from build123d import *

# Parameters (mm, degrees)
ESQUISSE1_R           = 9
BOSS_EXTRU_1_DEPTH    = 5
ESQUISSE1_R_2         = 25.075
ESQUISSE1_R_3         = 23.6
BOSS_EXTRU_1_2_DEPTH  = 5
ESQUISSE1_3_R         = 23.6
ESQUISSE1_3_R_2       = 9
BOSS_EXTRU_2_DEPTH    = 2
ESQUISSE1_4_R         = 29.5
ESQUISSE1_4_R_2       = 25.075
BOSS_EXTRU_3_DEPTH    = 5.1
CONG_1_R              = 2
CONG_1_OF_SYM_TRIE1_R = 2


with BuildPart() as part:
    # Esquisse1 → Boss.-Extru.1 (new body)
    with BuildSketch(Plane.XY):
        Circle(ESQUISSE1_R)
        with BuildLine():
            ThreePointArc((-3, 0), (2.001193394, -2.235), (0.33015, 2.981778157))
            Line((0.33015, 2.981778157), (-3, 0))
        make_face(mode=Mode.SUBTRACT)
    boss_extru_1 = extrude(amount=BOSS_EXTRU_1_DEPTH)



with BuildPart() as body_2:
    # Esquisse1 → Boss.-Extru.1 2 (new body)
    with BuildSketch(Plane.XY):
        Circle(ESQUISSE1_R_2)
        Circle(ESQUISSE1_R_3, mode=Mode.SUBTRACT)
    boss_extru_1_2 = extrude(amount=BOSS_EXTRU_1_2_DEPTH)


with BuildPart() as part_1:
    add(part.part)

    add(body_2.part)  # Boss.-Extru.2 merges body 2
    # Esquisse1<3> → Boss.-Extru.2 (add)
    with BuildSketch(Plane.XY):
        Circle(ESQUISSE1_3_R)
        Circle(ESQUISSE1_3_R_2, mode=Mode.SUBTRACT)
    boss_extru_2 = extrude(amount=BOSS_EXTRU_2_DEPTH)

    # Esquisse1<4> → Boss.-Extru.3 (add)
    with BuildSketch(Plane.XY):
        Circle(ESQUISSE1_4_R)
        Circle(ESQUISSE1_4_R_2, mode=Mode.SUBTRACT)
    boss_extru_3 = extrude(amount=BOSS_EXTRU_3_DEPTH)

    # Congé1
    cong_1_edges = [part_1.edges().sort_by_distance(p)[0] for p in [
        (-9, 0, 2),
        (-23.6, 0, 2),
    ]]
    fillet(cong_1_edges, radius=CONG_1_R)


with BuildPart() as sym_trie1_1:
    # Symétrie1: Boss.-Extru.1, Boss.-Extru.1 2, Boss.-Extru.2, Boss.-Extru.3 across Front Plane
    add(boss_extru_1.mirror(Plane.XY))
    add(boss_extru_1_2.mirror(Plane.XY))
    add(boss_extru_2.mirror(Plane.XY))
    add(boss_extru_3.mirror(Plane.XY))

    # Congé1 of Symétrie1
    cong_1_of_sym_trie1_edges = [sym_trie1_1.edges().sort_by_distance(p)[0] for p in [
        (-9, 0, -2),
        (-23.6, 0, -2),
    ]]
    fillet(cong_1_of_sym_trie1_edges, radius=CONG_1_OF_SYM_TRIE1_R)


with BuildPart() as part_2:
    add(part_1.part)

    # Symétrie1 united with what the copies to: union Symétrie1_1
    add(sym_trie1_1.part)


solid = part_2.part
Design review of the part built by this model. Coordinates are the model's own, in mm. A direction names the side the tool comes from. Coordinates: 2 decimals unless noted, no trailing zeros. Write each loop counter-clockwise with the first axis right and the second up, starting at its lowest first coordinate (ties: lowest second). Pieces come first, ordered by that corner, then holes. Notation, with made-up numbers: (23, -39.75) - (41, -39.75) arc R6 cw to (41, -32.75) - close; hole circle Ø3 at (-33, 55). An arc over 180 degrees is marked (long way). Use one line per item in the form item = value.
Q1. Consider section A-A (z = 3). Write out the cut boundary in (x, y), plus the area to 3 significant figures.
Taken from the geometry:
outline = circle Ø59 at (0, 0); circle Ø18.54 at (0, 0); hole circle Ø46.66 at (0, 0); hole (-3, 0) arc R3 ccw (long way) to (0.33, 2.98) - close
area = 1,270 mm^2
Q2. The part is to be moulded in two halves that separate along X. For faces 1 (the cylindrical face through (-1.172, 8.923, 4.493)), 2 (the flat face through (-10, 5, 2)), 3 (the flat face through (-13, -22, 5.1)), 4 (the cylindrical face through (28.14, 8.86, 0.07)), say which applies: +X half, -X half, draft (parallel to the pull), parting line (faces both ways), or undercut.
Taken from the geometry:
face_1 = undercut
face_2 = undercut
face_3 = draft
face_4 = parting line
Q3. Machinability: for faces 5 (the flat face through (17, 17, -5)), 6 (the flat face through (-2, 2, 5)), 7 (the flat face through (-13, -22, -5.1)), 8 (the flat face through (-1.312, 1.512, 0.07)), which of the approach directions +Z, -Z, +X, -X, +Y, -Y give a long, thin tool a straight path to every point of the face, cutting with its end or side? Answer none if there is none.
Taken from the geometry:
face_5 = -Z
face_6 = +Z
face_7 = -Z, +X, -X, +Y, -Y
face_8 = +Z, -Z
Q4. Insertion check: pin 1 Ø5 at (y, z) = (8, 3) entering from +X; pin 2 Ø9 at (x, y) = (3, 4) entering from -Z; pin 3 Ø1.5 at (y, z) = (-2, -2.5) entering from +X. Each pin has a flat end and moves straight along its axis. Give the tip position at first contact, or say it passes through.
Taken from the geometry:
pin_1 = 28.98
pin_2 = -5
pin_3 = 29.47
Q5. For probe 1 along Y at (x, z) = (0, -4.55); probe 2 along Y at (x, z) = (3.5, -3); probe 3 along X at (y, z) = (5, -3.75), list the stretches that pass through material, from the lowest coordinate up.
Taken from the geometry:
probe_1 = -29.5 to -23.6, -9 to -3, 2.69 to 9, 23.6 to 29.5
probe_2 = -29.29 to -23.07, -8.58 to 8.58, 23.07 to 29.29
probe_3 = -29.07 to -23.05, -7.5 to 7.5, 23.05 to 29.07
Q6. Consider section B-B (z = -0.5). Write out the cut boundary in (x, y).
Taken from the geometry:
outline = circle Ø59 at (0, 0); hole (-3, 0) arc R3 ccw (long way) to (0.33, 2.98) - close
